Geometry: final body of the model. Coordinates: model frame, mm. Face numbers are marked on the shaded views. A direction names the side the tool comes from. Give positions to 0.01 mm unless a question says otherwise; leave off trailing zeros. Order: outer loops, then holes, each group sorted by start corner. A loop starts at its lowest first (then second) coordinate and runs counter-clockwise, first axis right, second up. Notation, with made-up numbers: (64.25, 15.5) -> (87.25, 15.5) arc R12 cw to (87.25, 26.5) -> close; hole circle Ø5 at (5.25, -23). An arc over 180 degrees is marked (long way). Answer in a Markdown table with one row per item. Add a question column.
Q1. Line query: line 1 along Z through (x, y) = (-8.5, 14.5); line 2 along X through (y, z) = (20.3, 0); line 3 along Z through (x, y) = (8, 3.25). Output: solid intervals per line, ascending. Write a range as from..to.
Q2. Cut plane A-A on z = 0. Return the cut outline in (x, y).
Q3. Contact query for flat-ended pins moving along their axis: P1, Ø9, axis at x = 0, z = 0, coming from the +Y side; P2, Ø8, axis at x = 4.5, y = 3.5, coming from the +Z side; P3, Ø2, axis at y = 21.5, z = 2, coming from the +X side; P4, Ø5, axis at x = 7.5, y = 21.5, coming from the -Z side. Output: stop coordinate, or through.
Q4. Cut plane C-C on y = 9. Return the cut outline in (x, z), and give its area (3 significant figures).
Q5. Set-up query: the marked faces 5, 6 and 7. Return all of +Z, -Z, +X, -X, +Y, -Y with unobstructed straight access to the full face (end or side cutting, diameter ignored); none if empty.
Q6. Cut plane D-D on y = 3.75. Return the cut outline in (x, z), and give its area (3 significant figures).
Q7. Pull-direction query (X, two-part tool) for the marked faces 1, 2, 3 and 4; classes: +X half, -X half, draft (parallel to the pull), parting line (faces both ways), or undercut.
from build123d import *

# Parameters (mm, degrees)
REVOLVE1_ANGLE      = 230
SKETCH2_W           = 21
SKETCH2_H           = 10
BOSS_EXTRUDE1_DEPTH = 24
FILLET1_R           = 12
SKETCH3_R           = 4
CUT_EXTRUDE1_DEPTH  = 38.911080175


with BuildPart() as part:
    # Sketch1 → Revolve1 (revolve, symmetric)
    with BuildSketch(Plane(origin=(0, 0, 0), x_dir=(0, 0, -1), z_dir=(1, 0, 0))) as revolve1_sk:
        Polygon((10.5, 24), (7.5, 24), (7.5, 20.67), (7.2, 20.67), (7.2, 19.03), (7.5, 19.03), (7.5, 4.97), (7.2, 4.97), (7.2, 3.33), (7.5, 3.33), (7.5, 0), (10.5, 0), align=None)
    revolve(axis=Axis((0, -542.901644974, 0), (0, 1, 0)), revolution_arc=REVOLVE1_ANGLE / 2)
    revolve(revolve1_sk.sketch, axis=Axis((0, -542.901644974, 0), (0, -1, 0)), revolution_arc=REVOLVE1_ANGLE / 2)

    # Sketch2 → Boss-Extrude1 (add)
    with BuildSketch(Plane(origin=(0, 24, 0), x_dir=(1, 0, 0), z_dir=(0, 1, 0))):
        with Locations((0, 15.5)):
            Rectangle(SKETCH2_W, SKETCH2_H)
        with BuildLine():
            Line((10.5, 10.5), (1.4e-08, 10.5))
            ThreePointArc((1.4e-08, 10.5), (4.018176046, 9.700735089), (7.424621202, 7.424621202))
            Line((7.424621202, 7.424621202), (10.5, 10.5))
        make_face()
        with BuildLine():
            Line((1.4e-08, 10.5), (-10.5, 10.5))
            Line((-10.5, 10.5), (-7.424621202, 7.424621202))
            ThreePointArc((-7.424621202, 7.424621202), (-4.018176034, 9.700735094), (1.4e-08, 10.5))
        make_face()
    extrude(amount=-BOSS_EXTRUDE1_DEPTH)

    # Fillet1
    fillet1_edges = [part.edges().sort_by_distance(p)[0] for p in [
        (0, 0, -20.5),
        (0, 24, -20.5),
    ]]
    fillet(fillet1_edges, radius=FILLET1_R - 0.0001)  # a hair under: the kernel refuses the full size

    # Sketch3 → Cut-Extrude1 (cut, through all)
    with BuildSketch(Plane.ZY.offset(10.5)):
        with Locations((-14.5, 12)):
            Circle(SKETCH3_R)
    extrude(amount=-CUT_EXTRUDE1_DEPTH, mode=Mode.SUBTRACT)


solid = part.part
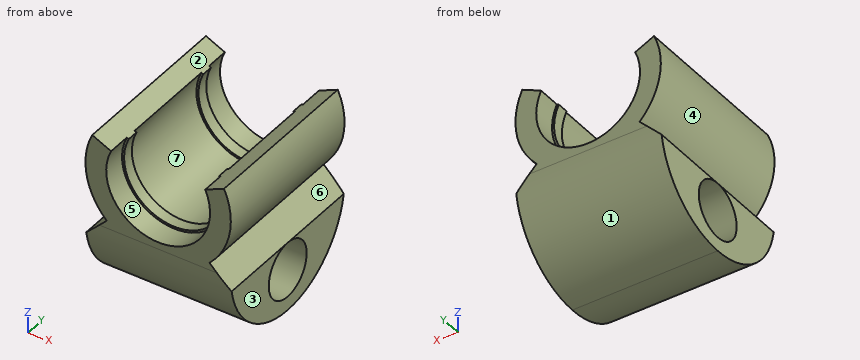
Completed:
| question | item | result |
|---|---|---|
| 1 | line 1 | z = -20.24..-17.62, -11.38..-8.5, -6.16..3.96 |
| 1 | line 2 | x = -10.5..-7.2, 7.2..10.5 |
| 1 | line 3 | z = -16.71..-8, -6.8..3.73 |
| 2 | outline | (-10.5, 0) -> (-7.5, 0) -> (-7.5, 3.33) -> (-7.2, 3.33) -> (-7.2, 4.97) -> (-7.5, 4.97) -> (-7.5, 19.03) -> (-7.2, 19.03) -> (-7.2, 20.67) -> (-7.5, 20.67) -> (-7.5, 24) -> (-10.5, 24) -> close; (7.2, 3.33) -> (7.5, 3.33) -> (7.5, 0) -> (10.5, 0) -> (10.5, 24) -> (7.5, 24) -> (7.5, 20.67) -> (7.2, 20.67) -> (7.2, 19.03) -> (7.5, 19.03) -> (7.5, 4.97) -> (7.2, 4.97) -> close |
| 3 | P1 | passes through |
| 3 | P2 | stops at z = 3.96 |
| 3 | P3 | stops at x = 10.45 |
| 3 | P4 | stops at z = -18.25 |
| 4 | outline | (-10.5, -20.12) -> (10.5, -20.12) -> (10.5, -17.15) -> (-10.5, -17.15) -> close; (-10.5, -11.85) -> (10.5, -11.85) -> (10.5, -10.5) -> (7.42, -7.42) arc R10.5 ccw to (9.52, 4.44) -> (6.8, 3.17) arc R7.5 cw (long way) to (-6.8, 3.17) -> (-9.52, 4.44) arc R10.5 ccw to (-7.42, -7.42) -> (-10.5, -10.5) -> close |
| 4 | area | 223 mm² |
| 5 | face 5 | -Y |
| 5 | face 6 | +X, +Y, -Y |
| 5 | face 7 | none |
| 6 | outline | (-10.5, -17.21) -> (10.5, -17.21) -> (10.5, -10.5) -> (7.42, -7.42) arc R10.5 ccw to (9.52, 4.44) -> (6.53, 3.04) arc R7.2 cw (long way) to (-6.53, 3.04) -> (-9.52, 4.44) arc R10.5 ccw to (-7.42, -7.42) -> (-10.5, -10.5) -> close |
| 6 | area | 282 mm² |
| 7 | face 1 | draft |
| 7 | face 2 | undercut |
| 7 | face 3 | +X half |
| 7 | face 4 | -X half |
